Here's the drawing with two shaded views (mm, measured from the low corner). I have some questions. A direction names the side the tool comes from. Coordinates: 2 decimals unless noted, no trailing zeros. Write each loop counter-clockwise with the first axis right and the second up, starting at its lowest first coordinate (ties: lowest second). Pieces come first, ordered by that corner, then holes. Notation, with made-up numbers: (32.5, 63.25) - (49.5, 63.25) arc R25 ccw to (49.5, 100.25) - close; hole circle Ø1 at (72.5, 71.25). An arc over 180 degrees is marked (long way). Answer in a Markdown table with one row per item. Add a question column.
Item 1: If I drill on probe 1 along Z at (x, y) = (4, 2); probe 2 along Y at (x, z) = (12.5, 12.5); probe 3 along X at (y, z) = (3.15, 20), over which ranges is the centre line in solid material (lowest first)? Write a range as from..to.
Item 2: Which directions (+Z, -Z, +X, -X, +Y, -Y) give clear straight access to the entire face, cutting with the end or side of a thin tool? Please do the marked faces 1 and 2.
Item 3: Imagine slicing it at D-D (z = 5). Please give me the cut outline in (x, y).
Item 4: Imagine slicing it at A-A (y = 2). Please give me the cut outline in (x, z).
Item 5: We'd pull the mould along X, two halves only. Please class the marked faces 3, 4 and 5: +X half, -X half, draft (parallel to the pull), parting line (faces both ways), or undercut.
Item 6: Imagine slicing it at C-C (x = 12.5). Please give me the cut outline in (y, z), plus the area to 3 significant figures.
Item 7: I'm going to push a flat-ended pin straight in: pin 1 (1.2 mm diameter, centred on y = 1, z = 5, fed in from +X). Where does the tip first touch, or does it pass through?
Item 8: Imagine slicing it at B-B (x = 4). Please give me the cut outline in (y, z), plus the area to 3 significant figures.
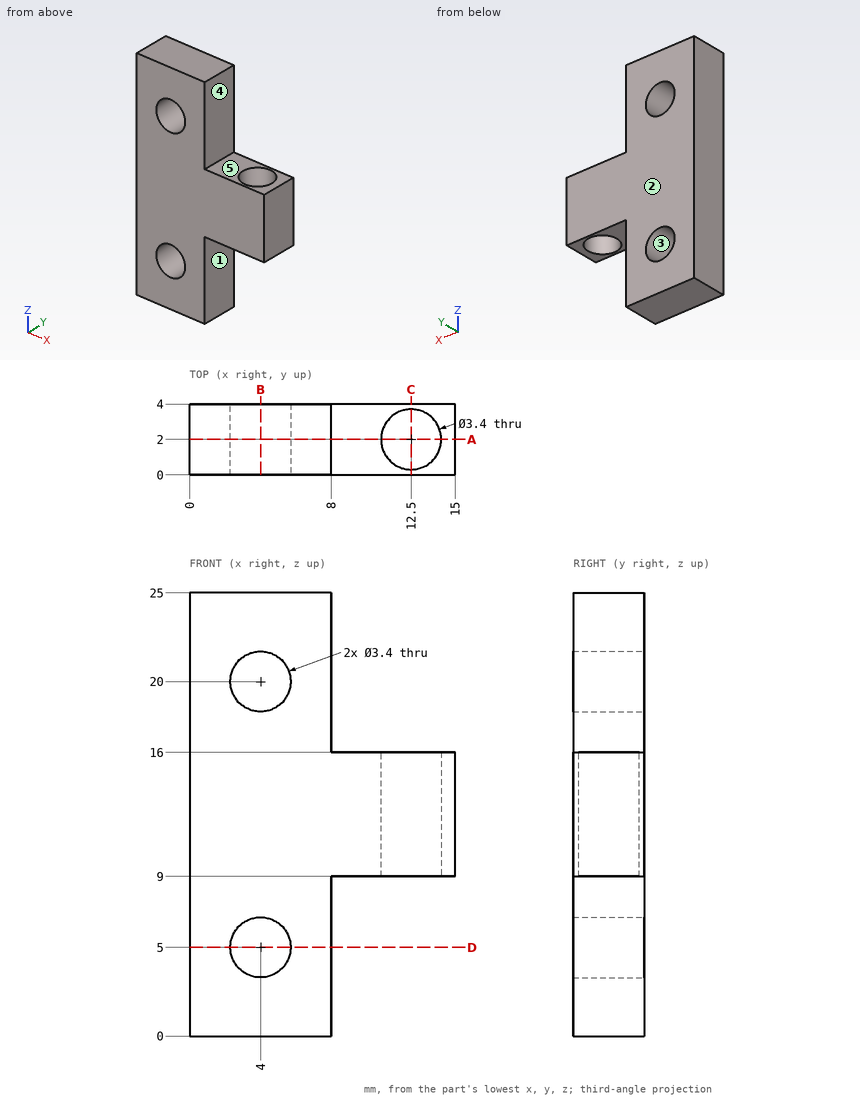
Here are the results:
| question | item | result |
|---|---|---|
| 1 | probe 1 | z = 0..3.3, 6.7..18.3, 21.7..25 |
| 1 | probe 2 | y = 0..0.3, 3.7..4 |
| 1 | probe 3 | x = 0..2.3, 5.7..8 |
| 2 | face 1 | -Z, +X, +Y, -Y |
| 2 | face 2 | +Z, -Z, +X, -X, +Y |
| 3 | outline | (0, 0) - (2.3, 0) - (2.3, 4) - (0, 4) - close; (5.7, 0) - (8, 0) - (8, 4) - (5.7, 4) - close |
| 4 | outline | (0, 0) - (8, 0) - (8, 9) - (10.8, 9) - (10.8, 16) - (8, 16) - (8, 25) - (0, 25) - close; (14.2, 9) - (15, 9) - (15, 16) - (14.2, 16) - close; hole circle Ø3.4 at (4, 5); hole circle Ø3.4 at (4, 20) |
| 5 | face 3 | undercut |
| 5 | face 4 | +X half |
| 5 | face 5 | draft |
| 6 | outline | (0, 9) - (0.3, 9) - (0.3, 16) - (0, 16) - close; (3.7, 9) - (4, 9) - (4, 16) - (3.7, 16) - close |
| 6 | area | 4.20 mm2 |
| 7 | pin 1 | stops at x = 8 |
| 8 | outline | (0, 0) - (4, 0) - (4, 3.3) - (0, 3.3) - close; (0, 6.7) - (4, 6.7) - (4, 18.3) - (0, 18.3) - close; (0, 21.7) - (4, 21.7) - (4, 25) - (0, 25) - close |
| 8 | area | 72.8 mm2 |
